from build123d import *

# Parameters (mm, degrees)
SKETCH1_W               = 22.225
SKETCH1_H               = 22.225
BOSS_EXTRUDE1_DEPTH     = 23.8125
F_1_4_CLEARANCE_HOLE1_D = 6.7564
CHAMFER1_SIZE           = 1.524


with BuildPart() as part:
    # Sketch1 → Boss-Extrude1 (new, symmetric)
    with BuildSketch(Plane.XY):
        Rectangle(SKETCH1_W, SKETCH1_H)
    extrude(amount=BOSS_EXTRUDE1_DEPTH, both=True)

    # 1/4 Clearance Hole1 (through all)
    with Locations(Plane(origin=(0, 11.1125, 0), x_dir=(1, 0, 0), z_dir=(0, 1, 0))):
        with Locations((0, 15.875), (0, -15.875), (0, 0)):
            Hole(F_1_4_CLEARANCE_HOLE1_D / 2)

    # Chamfer1
    chamfer1_edges = [part.edges().sort_by_distance(p)[0] for p in [
        (11.1125, 0, 23.8125),
        (0, 11.1125, 23.8125),
        (-11.1125, 0, 23.8125),
        (0, 11.1125, -23.8125),
        (11.1125, 0, -23.8125),
        (0, -11.1125, -23.8125),
        (-11.1125, 0, -23.8125),
        (-11.1125, 11.1125, 0),
        (11.1125, 11.1125, 0),
        (11.1125, -11.1125, 0),
        (-11.1125, -11.1125, 0),
        (0, -11.1125, 23.8125),
    ]]
    chamfer(chamfer1_edges, length=CHAMFER1_SIZE)


solid = part.part
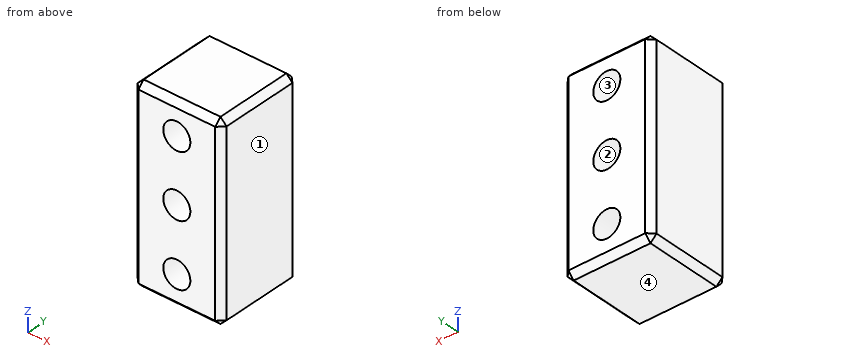
For this review, take the finished solid that the model builds, in its own axes (mm). Face numbers are marked on the shaded views. Round coordinates to 2 decimals unless told otherwise and drop trailing zeros. Order: outer loops, then holes, each group sorted by start corner. A loop starts at its lowest first (then second) coordinate and runs counter-clockwise, first axis right, second up. Notation, with made-up numbers: M -28.5,56 L 28.5,56 A18 cw 28.5,78 Z; hole C 34.5,-26 d9. An arc over 180 degrees is marked long. Write each question's results on one line, items separated by ' | '. Start each with the question number.
1. Add section A-A (z = 0). State the section outline as (x, y) points, then the cut area to 3 significant figures.
2. To check wall thickness, follow L1, parallel to Z at x = 0, y = -3; L2, parallel to X at y = -9.5, z = -16; L3, parallel to Z at x = 2.5, y = -10. State the ranges of each line that lie inside material, in increasing order. Write a range as [from, to].
3. Draft analysis for pull direction X (two halves, no side actions). For the marked faces 1, 2, 3 and 4, state which applies: pulls with the +X half, pulls with the -X half, needs draft (parallel to the pull), parting line crosses it, or undercut.
4. Add section B-B (x = 0). State the section outline as (y, z) points.
5. Add section C-C (y = -0.5). State the section outline as (x, z) points (1 decimal).
Output values:
1) outline: M -11.11,-9.59 L -9.59,-11.11 L -3.38,-11.11 L -3.38,11.11 L -9.59,11.11 L -11.11,9.59 Z; M 3.38,-11.11 L 9.59,-11.11 L 11.11,-9.59 L 11.11,9.59 L 9.59,11.11 L 3.38,11.11 Z | area: 339 mm^2
2) L1: [-23.81, -19.25], [-12.5, -3.38], [3.38, 12.5], [19.25, 23.81] | L2: [-11.11, -3.38], [3.38, 11.11] | L3: [-23.4, -18.15], [-13.6, -2.27], [2.27, 13.6], [18.15, 23.4]
3) face 1: pulls with the +X half | face 2: undercut | face 3: undercut | face 4: needs draft
4) outline: M -11.11,-22.29 L -9.59,-23.81 L 9.59,-23.81 L 11.11,-22.29 L 11.11,-19.25 L -11.11,-19.25 Z; M -11.11,-12.5 L 11.11,-12.5 L 11.11,-3.38 L -11.11,-3.38 Z; M -11.11,3.38 L 11.11,3.38 L 11.11,12.5 L -11.11,12.5 Z; M -11.11,19.25 L 11.11,19.25 L 11.11,22.29 L 9.59,23.81 L -9.59,23.81 L -11.11,22.29 Z
5) outline: M -11.1,-22.3 L -9.6,-23.8 L 9.6,-23.8 L 11.1,-22.3 L 11.1,22.3 L 9.6,23.8 L -9.6,23.8 L -11.1,22.3 Z; hole C 0,-15.9 d6.8; hole C 0,0 d6.8; hole C 0,15.9 d6.8
